Geometry check sheet. Reference: drawing and pictorial views, mm from the part's lowest x, y, z. A direction names the side the tool comes from. Give positions to 0.01 mm unless a question says otherwise; leave off trailing zeros. Loops run counter-clockwise (first coordinate to the right, second up) from the corner with the lowest first, then second, coordinate; pieces in that order, holes last. Notation, with made-up numbers: (30.5, 27) -> (43.5, 27) arc R21 cw to (43.5, 40) -> close; hole circle Ø10 at (1, -24.75). An arc over 180 degrees is marked (long way). Write each question's results on one line, items separated by ' | '. Start each with the question number.
1. Cross-section at A-A on x = 10. Record the boundary of the cut face in (y, z), and give its area (3 significant figures).
2. Mould release check, pull along X, two halves, no side actions. Record for the marked faces 3, 4 and 5: +X half, -X half, draft (parallel to the pull), parting line (faces both ways), or undercut.
3. Tool access check on the marked faces 1 and 2. Record the directions out of +Z, -Z, +X, -X, +Y, -Y that give a thin tool (end or side, any length) a straight path to the whole face; none if there is none.
4. Material ranges on L1, parallel to Y at x = 10, z = 16.25; L2, parallel to Z at x = 7.5, y = 11.5; L3, parallel to X at y = 9.75, z = 4.25, recorded low to high. Write a range as from..to.
5. Cross-section at C-C on z = 15. Record the boundary of the cut face in (x, y), and give its area (3 significant figures).
6. Gauge pin test, flat ends, axial feed: pin 1 Ø6 at (x, z) = (13, 16) entering from -Y; pin 2 Ø5 at (y, z) = (16, 2.5) entering from +X; pin 3 Ø3 at (y, z) = (16, 9.5) entering from -X; pin 4 Ø2 at (y, z) = (2, 12.5) entering from -X. Record the tip position at first contact, or that the pin passes through.
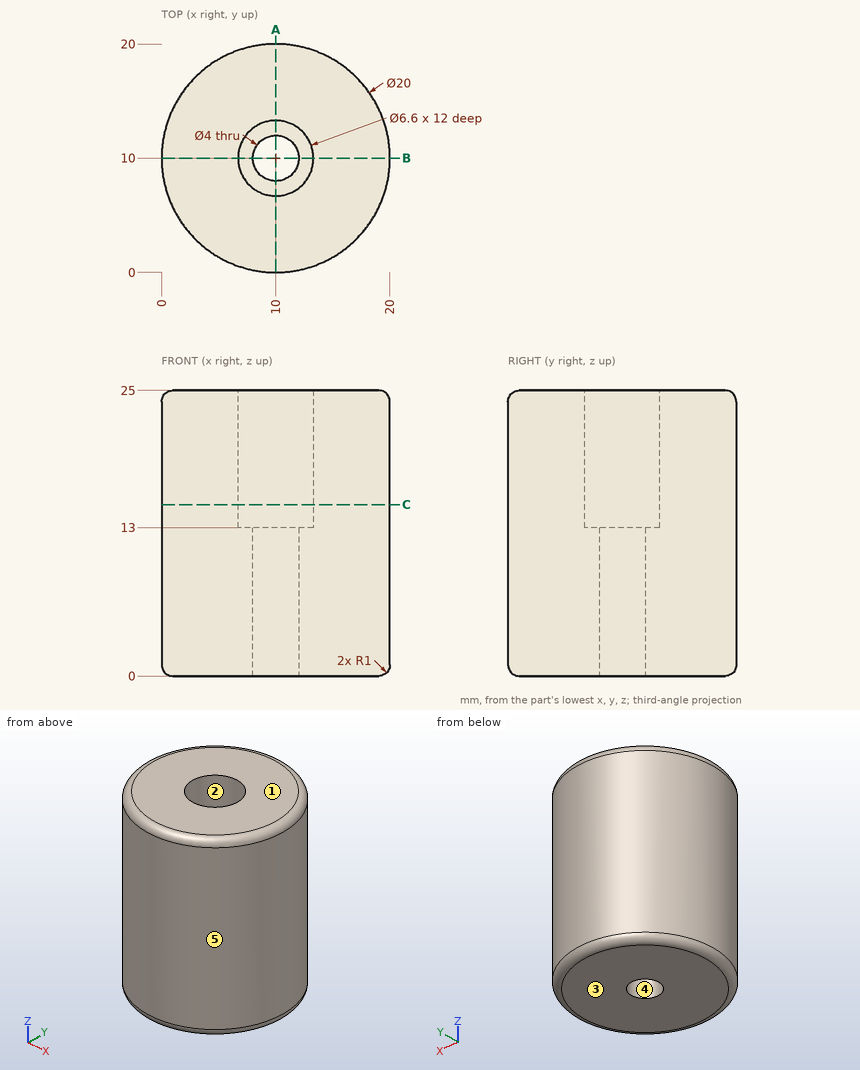
Geometry says:
1) outline: (0, 1) arc R1 ccw to (1, 0) -> (8, 0) -> (8, 13) -> (6.7, 13) -> (6.7, 25) -> (1, 25) arc R1 ccw to (0, 24) -> close; (12, 0) -> (19, 0) arc R1 ccw to (20, 1) -> (20, 24) arc R1 ccw to (19, 25) -> (13.3, 25) -> (13.3, 13) -> (12, 13) -> close | area: 368 mm^2
2) face 3: draft | face 4: undercut | face 5: parting line
3) face 1: +Z, +X, -X, +Y, -Y | face 2: +Z
4) L1: 0..6.7, 13.3..20 | L2: 0..13 | L3: 0..8.02, 11.98..20
5) outline: circle Ø20 at (10, 10); hole circle Ø6.6 at (10, 10) | area: 280 mm^2
6) pin 1: y = 0 | pin 2: x = 19.37 | pin 3: x = 1.07 | pin 4: x = 2.86
